The listing builds one solid part. Answer for the finished solid, in the listing's coordinates (mm). A direction names the side the tool comes from. Give positions to 0.01 mm unless a question says otherwise; leave off trailing zeros. Order: outer loops, then holes, each group sorted by start corner. A loop starts at its lowest first (then second) coordinate and runs counter-clockwise, first axis right, second up. Notation, with made-up numbers: (19.25, -0.75) -> (34.25, -0.75) arc R9 ccw to (34.25, 4.25) -> close; hole circle Ø8 at (34, 56). An arc over 180 degrees is marked (long way). One line per question, with ' | ' between items. Start each with the question number.
```python
from build123d import *

# Parameters (mm, degrees)
SKETCH1_R           = 1.5
BOSS_EXTRUDE1_DEPTH = 1.5


with BuildPart() as part:
    # Sketch1 → Boss-Extrude1 (new body)
    with BuildSketch(Plane(origin=(0, 0, 0), x_dir=(1, 0, 0), z_dir=(0, 1, 0))):
        with BuildLine():
            Line((-8.464101615, -2), (-13.660254038, -5))
            ThreePointArc((-13.660254038, -5), (-14.758330249, -9.098076211), (-10.660254038, -10.196152423))
            Line((-10.660254038, -10.196152423), (-5.464101615, -7.196152423))
            Line((-5.464101615, -7.196152423), (-1.464101615, -7.196152423))
            Line((-1.464101615, -7.196152423), (3.732050808, -10.196152423))
            ThreePointArc((3.732050808, -10.196152423), (7.830127019, -9.098076211), (6.732050808, -5))
            Line((6.732050808, -5), (1.535898385, -2))
            Line((1.535898385, -2), (-8.464101615, -2))
        make_face()
        with Locations(Location((-12.160254038, -7.598076211, 0), (0, 0, 270))):
            Circle(SKETCH1_R, mode=Mode.SUBTRACT)
        with Locations(Location((5.232050808, -7.598076211, 0), (0, 0, 90))):
            Circle(SKETCH1_R, mode=Mode.SUBTRACT)
    extrude(amount=BOSS_EXTRUDE1_DEPTH)


solid = part.part
```
(1) The part is cut by section B-B on z = 8. Determine the outline of the cut face in (x, y) (3 decimals).
(2) Consider line 1 (X direction, y = 0.7, z = 7.25); line 2 (X direction, y = 0.4, z = 8) (3 decimals); line 3 (Z direction, x = -2.25, y = 0.2). Determine where each line is inside the solid, lowest interval first.
(3) The part is cut by section C-C on x = 6.5. Determine the outline of the cut face in (y, z).
(4) The part is cut by section A-A on y = 0.7. Determine the outline of the cut face in (x, z).
(5) Determine the mould class of faces 1 (the face through (7.8, 0.74, 9.15)), 2 (the face through (-12.735, 0.74, 8.984)), 3 (the face through (4.17, 0.74, 3.52)) for opening direction Z: pulls with the +Z half, pulls with the -Z half, needs draft (parallel to the pull), parting line crosses it, or undercut.
(6) For faces 4 (the face through (-8.1, 0.74, 8.72)), 5 (the face through (-4, 0, 6)), determine the directions among +Z, -Z, +X, -X, +Y, -Y from which every point of the face is accessible in a straight line to the end or side of a thin tool.
(7) The part is cut by section D-D on z = 9.5. Determine the outline of the cut face in (x, y).
(8) Given P1, Ø5, axis at x = -3, z = 6.5, coming from the -Y side, flat-ended and moving along its own axis, determine where the tip first touches the part or whether it passes through.
Result sheet:
1) outline: (-15.133, 0) -> (-13.605, 0) -> (-13.605, 1.5) -> (-15.133, 1.5) -> close; (-10.715, 0) -> (-6.856, 0) -> (-6.856, 1.5) -> (-10.715, 1.5) -> close; (-0.072, 0) -> (3.787, 0) -> (3.787, 1.5) -> (-0.072, 1.5) -> close; (6.677, 0) -> (8.205, 0) -> (8.205, 1.5) -> (6.677, 1.5) -> close
2) line 1: x = -15.14 to -13.62, -10.7 to -5.56, -1.37 to 3.77, 6.69 to 8.21 | line 2: x = -15.133 to -13.605, -10.715 to -6.856, -0.072 to 3.787, 6.677 to 8.205 | line 3: z = 2 to 7.2
3) outline: (0, 4.87) -> (1.5, 4.87) -> (1.5, 6.8) -> (0, 6.8) -> close; (0, 8.4) -> (1.5, 8.4) -> (1.5, 10.32) -> (0, 10.32) -> close
4) outline: (-13.66, 5) -> (-8.46, 2) -> (1.54, 2) -> (6.73, 5) arc R3 ccw to (3.73, 10.2) -> (-1.46, 7.2) -> (-5.46, 7.2) -> (-10.66, 10.2) arc R3 ccw to start; hole circle Ø3 at (-12.16, 7.6); hole circle Ø3 at (5.23, 7.6)
5) face 1: parting line crosses it | face 2: undercut | face 3: pulls with the -Z half
6) face 4: +Z, +Y, -Y | face 5: +Z, -Z, +X, -X, -Y
7) outline: (-14.48, 0) -> (-9.45, 0) -> (-9.45, 1.5) -> (-14.48, 1.5) -> close; (2.53, 0) -> (7.55, 0) -> (7.55, 1.5) -> (2.53, 1.5) -> close
8) P1: stops at y = 0
